Design review of the part built by this model. Coordinates are the model's own, in mm. A direction names the side the tool comes from. Coordinates: 2 decimals unless noted, no trailing zeros. Loops run counter-clockwise (first coordinate to the right, second up) from the corner with the lowest first, then second, coordinate; pieces in that order, holes last. Notation, with made-up numbers: M 87,-7 L 95,-7 A31 ccw 95,22 Z; hole C 53,48 d3. An arc over 180 degrees is marked long. Put each result on its own line as item: value. Start each with the question number.
(1) The part is to be moulded in two halves that separate along X. For faces 3 (the flat face through (-298, -5, 10)), 4 (the flat face through (-290, 2, 20)), 5 (the flat face through (300, -5, 10)), say which applies: +X half, -X half, draft (parallel to the pull), parting line (faces both ways), or undercut.
(2) Take a section at C-C, the plane y = -50. Give the boundary of the cut face in (x, z).
(3) For faces 1 (the flat face through (-4, -384, 10)), 2 (the flat face through (298, -5, 10)), list the 3-axis set-ups (+Z, -Z, +X, -X, +Y, -Y) from which the entire face can be reached by the end or side of a thin tool; tool diameter is ignored.
(4) Clearance check with a flat-ended pin moving along its axis: pin 1 (1 mm diameter, centred on x = -189, y = 43, fed in from +Z). State where the tip first meets the part, or that it passes through.
(5) Take a section at B-B, the plane x = 124.5. Give the boundary of the cut face in (y, z), then the cut area to 3 significant figures.
(6) For probe 1 along X at (y, z) = (-109, 3); probe 2 along Y at (x, z) = (-19, 15.5); probe 3 along Z at (x, y) = (116, 65), list the stretches that pass through material, from the lowest coordinate up. Write a range as [from, to].
(7) Take a section at A-A, the plane z = 14.75. Give the boundary of the cut face in (x, y).
```python
from build123d import *

# Parameters (mm, degrees)
SKETCH1_W           = 600
SKETCH1_H           = 768
BOSS_EXTRUDE1_DEPTH = 20
SHELL1_T            = -2
SKETCH2_W           = 596
SKETCH2_H           = 764
SKETCH2_W_2         = 566
SKETCH2_H_2         = 734
BOSS_EXTRUDE2_DEPTH = 2


with BuildPart() as part:
    # Sketch1 → Boss-Extrude1 (new body)
    with BuildSketch(Plane.XY):
        Rectangle(SKETCH1_W, SKETCH1_H)
    extrude(amount=BOSS_EXTRUDE1_DEPTH)

    # Shell1
    shell1_openings = [part.faces().sort_by_distance(p)[0] for p in [
        (0, 0, 20),
    ]]
    offset(amount=SHELL1_T, openings=shell1_openings, kind=Kind.INTERSECTION)

    # Sketch2 → Boss-Extrude2 (add)
    with BuildSketch(Plane.XY.offset(20)):
        Rectangle(SKETCH2_W, SKETCH2_H)
        Rectangle(SKETCH2_W_2, SKETCH2_H_2, mode=Mode.SUBTRACT)
    extrude(amount=-BOSS_EXTRUDE2_DEPTH)


solid = part.part
```
Computed values:
1. face 3: undercut
1. face 4: draft
1. face 5: +X half
2. outline: M -300,0 L 300,0 L 300,20 L 283,20 L 283,18 L 298,18 L 298,2 L -298,2 L -298,18 L -283,18 L -283,20 L -300,20 Z
3. face 1: +Z, -Z, +X, -X, -Y
3. face 2: none
4. pin 1: stops at z = 2
5. outline: M -384,0 L 384,0 L 384,20 L 367,20 L 367,18 L 382,18 L 382,2 L -382,2 L -382,18 L -367,18 L -367,20 L -384,20 Z
5. area: 1,670 mm^2
6. probe 1: x = [-300, -298], [298, 300]
6. probe 2: y = [-384, -382], [382, 384]
6. probe 3: z = [0, 2]
7. outline: M -300,-384 L 300,-384 L 300,384 L -300,384 Z; hole M -298,-382 L 298,-382 L 298,382 L -298,382 Z
